Verification items for the finished model (mm, model axes). Round coordinates to 2 decimals unless told otherwise and drop trailing zeros. Order: outer loops, then holes, each group sorted by start corner. A loop starts at its lowest first (then second) coordinate and runs counter-clockwise, first axis right, second up. Notation, with made-up numbers: (66.25, -1) -> (84.25, -1) arc R15 cw to (84.25, 23) -> close; hole circle Ø9 at (-6.75, -36). An arc over 180 degrees is marked (long way). Return JSON: item names as keys, results as strings. Group by question number.
1) Section check B-B on x = 0. Enter the section's corners in (y, z), plus the area to 3 significant figures.
2) Scan lines: L1, parallel to Y at x = 0, z = -82; L2, parallel to Y at x = 6.5, z = -36.5; L3, parallel to X at y = -0.25, z = -59. Record each from-to range of solid material in increasing order.
3) Section check A-A on y = 0. Enter the section's corners in (x, z), plus the area to 3 significant figures.
4) Depth check by flat-ended pin: pin 1 (1 mm diameter, centred on y = -1.5, z = -59.5, fed in from +X); pin 2 (3 mm diameter, centred on y = -2, z = -91, fed in from -X); pin 3 (1.7 mm diameter, centred on x = 0.5, z = -47.5, fed in from +Y). Enter the tip coordinate at first touch or a pass-through.
```python
from build123d import *

# Parameters (mm, degrees)
SKETCH1_R      = 2.6035
EXTRUDE1_DEPTH = 102.87


with BuildPart() as part:
    # Sketch1 → Extrude1 (new body)
    with BuildSketch(Plane.XY):
        with BuildLine():
            Line((-1.709253557, -4.4958), (1.709253557, -4.4958))
            ThreePointArc((1.709253557, -4.4958), (2.922935876, -4.736928798), (3.95226937, -5.423689619))
            Line((3.95226937, -5.423689619), (7.179652728, -8.645192207))
            ThreePointArc((7.179652728, -8.645192207), (7.414733441, -9.822812921), (6.41641086, -10.4902))
            Line((6.41641086, -10.4902), (4.28752, -10.4902))
            ThreePointArc((4.28752, -10.4902), (3.545750844, -10.797450844), (3.2385, -11.53922))
            Line((3.2385, -11.53922), (3.2385, -11.65098))
            ThreePointArc((3.2385, -11.65098), (3.545750844, -12.392749156), (4.28752, -12.7))
            Line((4.28752, -12.7), (5.3171344, -12.7))
            ThreePointArc((5.3171344, -12.7), (5.8251344, -12.192), (6.3331344, -12.7))
            Line((6.3331344, -12.7), (9.5504, -12.7))
            ThreePointArc((9.5504, -12.7), (10.058323491, -12.192000006), (10.566399977, -12.699846982))
            ThreePointArc((10.566399977, -12.699846982), (12.082522516, -12.082522516), (12.699846982, -10.566399977))
            ThreePointArc((12.699846982, -10.566399977), (12.192000006, -10.058323491), (12.7, -9.5504))
            Line((12.7, -9.5504), (12.7, -6.3330836))
            ThreePointArc((12.7, -6.3330836), (12.192, -5.8250836), (12.7, -5.3170836))
            Line((12.7, -5.3170836), (12.7, -4.287470133))
            ThreePointArc((12.7, -4.287470133), (12.392749156, -3.545700977), (11.65098, -3.238450133))
            Line((11.65098, -3.238450133), (11.53922, -3.238450133))
            ThreePointArc((11.53922, -3.238450133), (10.797450844, -3.545700977), (10.4902, -4.287470133))
            Line((10.4902, -4.287470133), (10.4902, -6.402089023))
            ThreePointArc((10.4902, -6.402089023), (9.856394933, -7.351113629), (8.736962546, -7.129240479))
            Line((8.736962546, -7.129240479), (5.440484187, -3.838768792))
            ThreePointArc((5.440484187, -3.838768792), (4.75073678, -2.808015636), (4.5085, -1.591658411))
            Line((4.5085, -1.591658411), (4.5085, 1.591658411))
            ThreePointArc((4.5085, 1.591658411), (4.75073678, 2.808015636), (5.440484187, 3.838768792))
            Line((5.440484187, 3.838768792), (8.736962546, 7.129240479))
            ThreePointArc((8.736962546, 7.129240479), (9.856394933, 7.351113629), (10.4902, 6.402089023))
            Line((10.4902, 6.402089023), (10.4902, 4.287470133))
            ThreePointArc((10.4902, 4.287470133), (10.797450844, 3.545700977), (11.53922, 3.238450133))
            Line((11.53922, 3.238450133), (11.65098, 3.238450133))
            ThreePointArc((11.65098, 3.238450133), (12.392749156, 3.545700977), (12.7, 4.287470133))
            Line((12.7, 4.287470133), (12.7, 5.3171344))
            ThreePointArc((12.7, 5.3171344), (12.192, 5.8251344), (12.7, 6.3331344))
            Line((12.7, 6.3331344), (12.7, 9.5504))
            ThreePointArc((12.7, 9.5504), (12.192000006, 10.058323491), (12.699846982, 10.566399977))
            ThreePointArc((12.699846982, 10.566399977), (12.082522516, 12.082522516), (10.566399977, 12.699846982))
            ThreePointArc((10.566399977, 12.699846982), (10.058323491, 12.192000006), (9.5504, 12.7))
            Line((9.5504, 12.7), (6.3330836, 12.7))
            ThreePointArc((6.3330836, 12.7), (5.8250836, 12.192), (5.3170836, 12.7))
            Line((5.3170836, 12.7), (4.2874692, 12.7))
            ThreePointArc((4.2874692, 12.7), (3.545700044, 12.392749156), (3.2384492, 11.65098))
            Line((3.2384492, 11.65098), (3.2384492, 11.53922))
            ThreePointArc((3.2384492, 11.53922), (3.545700044, 10.797450844), (4.2874692, 10.4902))
            Line((4.2874692, 10.4902), (6.476774195, 10.4902))
            ThreePointArc((6.476774195, 10.4902), (7.43216212, 9.851515102), (7.207191475, 8.724540082))
            Line((7.207191475, 8.724540082), (3.900315394, 5.423689619))
            ThreePointArc((3.900315394, 5.423689619), (2.8709819, 4.736928798), (1.657299581, 4.4958))
            Line((1.657299581, 4.4958), (-1.657299581, 4.4958))
            ThreePointArc((-1.657299581, 4.4958), (-2.8709819, 4.736928798), (-3.900315394, 5.423689619))
            Line((-3.900315394, 5.423689619), (-7.207191475, 8.724540082))
            ThreePointArc((-7.207191475, 8.724540082), (-7.43216212, 9.851515102), (-6.476774195, 10.4902))
            Line((-6.476774195, 10.4902), (-4.2874692, 10.4902))
            ThreePointArc((-4.2874692, 10.4902), (-3.545700044, 10.797450844), (-3.2384492, 11.53922))
            Line((-3.2384492, 11.53922), (-3.2384492, 11.65098))
            ThreePointArc((-3.2384492, 11.65098), (-3.545700044, 12.392749156), (-4.2874692, 12.7))
            Line((-4.2874692, 12.7), (-5.3170836, 12.7))
            ThreePointArc((-5.3170836, 12.7), (-5.8250836, 12.192), (-6.3330836, 12.7))
            Line((-6.3330836, 12.7), (-9.5504, 12.7))
            ThreePointArc((-9.5504, 12.7), (-10.058323491, 12.192000006), (-10.566399977, 12.699846982))
            ThreePointArc((-10.566399977, 12.699846982), (-12.082522516, 12.082522516), (-12.699846982, 10.566399977))
            ThreePointArc((-12.699846982, 10.566399977), (-12.192000006, 10.058323491), (-12.7, 9.5504))
            Line((-12.7, 9.5504), (-12.7, 6.3331344))
            ThreePointArc((-12.7, 6.3331344), (-12.192, 5.8251344), (-12.7, 5.3171344))
            Line((-12.7, 5.3171344), (-12.7, 4.287470133))
            ThreePointArc((-12.7, 4.287470133), (-12.392749156, 3.545700977), (-11.65098, 3.238450133))
            Line((-11.65098, 3.238450133), (-11.53922, 3.238450133))
            ThreePointArc((-11.53922, 3.238450133), (-10.797450844, 3.545700977), (-10.4902, 4.287470133))
            Line((-10.4902, 4.287470133), (-10.4902, 6.402089023))
            ThreePointArc((-10.4902, 6.402089023), (-9.856394933, 7.351113629), (-8.736962546, 7.129240479))
            Line((-8.736962546, 7.129240479), (-5.440484187, 3.838768792))
            ThreePointArc((-5.440484187, 3.838768792), (-4.75073678, 2.808015636), (-4.5085, 1.591658411))
            Line((-4.5085, 1.591658411), (-4.5085, -1.591658411))
            ThreePointArc((-4.5085, -1.591658411), (-4.75073678, -2.808015636), (-5.440484187, -3.838768792))
            Line((-5.440484187, -3.838768792), (-8.736962546, -7.129240479))
            ThreePointArc((-8.736962546, -7.129240479), (-9.856394933, -7.351113629), (-10.4902, -6.402089023))
            Line((-10.4902, -6.402089023), (-10.4902, -4.287470133))
            ThreePointArc((-10.4902, -4.287470133), (-10.797450844, -3.545700977), (-11.53922, -3.238450133))
            Line((-11.53922, -3.238450133), (-11.65098, -3.238450133))
            ThreePointArc((-11.65098, -3.238450133), (-12.392749156, -3.545700977), (-12.7, -4.287470133))
            Line((-12.7, -4.287470133), (-12.7, -5.3170836))
            ThreePointArc((-12.7, -5.3170836), (-12.192, -5.8250836), (-12.7, -6.3330836))
            Line((-12.7, -6.3330836), (-12.7, -9.5504))
            ThreePointArc((-12.7, -9.5504), (-12.192000006, -10.058323491), (-12.699846982, -10.566399977))
            ThreePointArc((-12.699846982, -10.566399977), (-12.082522516, -12.082522516), (-10.566399977, -12.699846982))
            ThreePointArc((-10.566399977, -12.699846982), (-10.058323491, -12.192000006), (-9.5504, -12.7))
            Line((-9.5504, -12.7), (-6.3331344, -12.7))
            ThreePointArc((-6.3331344, -12.7), (-5.8251344, -12.192), (-5.3171344, -12.7))
            Line((-5.3171344, -12.7), (-4.28752, -12.7))
            ThreePointArc((-4.28752, -12.7), (-3.545750844, -12.392749156), (-3.2385, -11.65098))
            Line((-3.2385, -11.65098), (-3.2385, -11.53922))
            ThreePointArc((-3.2385, -11.53922), (-3.545750844, -10.797450844), (-4.28752, -10.4902))
            Line((-4.28752, -10.4902), (-6.41641086, -10.4902))
            ThreePointArc((-6.41641086, -10.4902), (-7.414733441, -9.822812921), (-7.179652728, -8.645192207))
            Line((-7.179652728, -8.645192207), (-3.95226937, -5.423689619))
            ThreePointArc((-3.95226937, -5.423689619), (-2.922935876, -4.736928798), (-1.709253557, -4.4958))
        make_face()
        Circle(SKETCH1_R, mode=Mode.SUBTRACT)
    extrude(amount=-EXTRUDE1_DEPTH)


solid = part.part
```
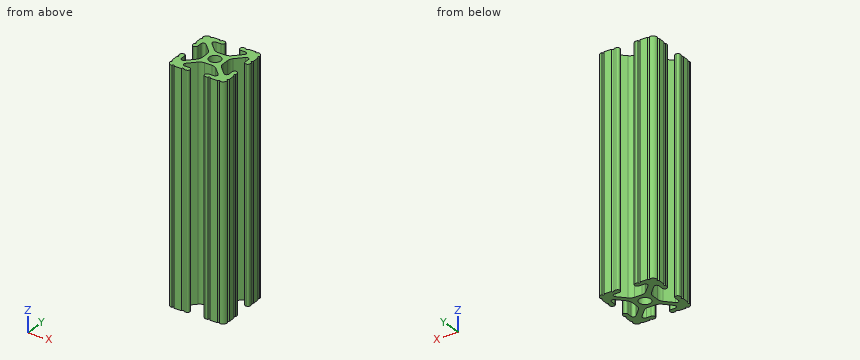
Check result:
{
 "1": {"outline": "(-4.5, -102.87) -> (-2.6, -102.87) -> (-2.6, 0) -> (-4.5, 0) -> close; (2.6, -102.87) -> (4.5, -102.87) -> (4.5, 0) -> (2.6, 0) -> close", "area": "389 mm^2"},
 "2": {"L1": "-4.5 to -2.6, 2.6 to 4.5", "L2": "-12.7 to -10.49, -7.97 to -4.9, 4.9 to 8.02, 10.49 to 12.7", "L3": "-4.51 to -2.59, 2.59 to 4.51"},
 "3": {"outline": "(-4.51, -102.87) -> (-2.6, -102.87) -> (-2.6, 0) -> (-4.51, 0) -> close; (2.6, -102.87) -> (4.51, -102.87) -> (4.51, 0) -> (2.6, 0) -> close", "area": "392 mm^2"},
 "4": {"pin 1": "x = 4.53", "pin 2": "x = -12.34", "pin 3": "y = 4.5"}
}
